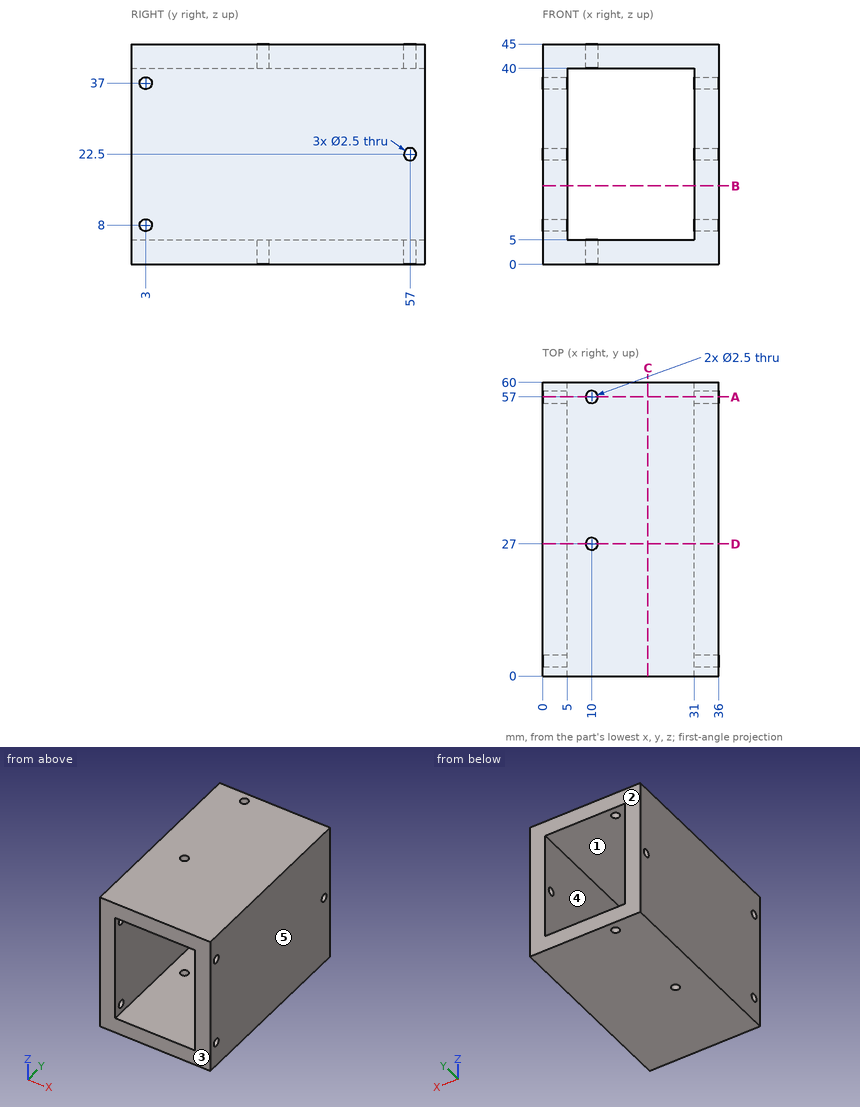
Here's the drawing with two shaded views (mm, measured from the low corner). I have some questions. A direction names the side the tool comes from. Give positions to 0.01 mm unless a question says otherwise; leave off trailing zeros. Order: outer loops, then holes, each group sorted by start corner. A loop starts at its lowest first (then second) coordinate and runs counter-clockwise, first axis right, second up.
Q1. If I drill on line 1 along X through (y, z) = (8, 9); line 2 along Z through (x, y) = (23, 24); line 3 along Y through (x, z) = (34, 8), over which ranges is the centre line in solid material (lowest first)?
Q2. We'd pull the mould along X, two halves only. Please class the marked faces 3, 4 and 5: +X half, -X half, draft (parallel to the pull), parting line (faces both ways), or undercut.
Q3. I'm going to push a flat-ended pin straight in: P1, Ø2, axis at y = 3, z = 37, coming from the -X side. Where does the tip first touch, or does it pass through?
Q4. Suppose I cut it at D-D, the plane y = 27. Write out the boundary of the cut face in (x, z), and give its area (3 significant figures).
Q5. For the marked faces 1 and 2, which set-ups out of +Z, -Z, +X, -X, +Y, -Y let a thin tool reach every point of the face, with its end or its side?
Q6. Suppose I cut it at C-C, the plane x = 21.5. Write out the boundary of the cut face in (y, z), and give its area (3 significant figures).
Q7. Suppose I cut it at B-B, the plane z = 16. Write out the boundary of the cut face in (x, y).
Q8. Suppose I cut it at A-A, the plane y = 57. Write out the boundary of the cut face in (x, z).
Solution:
1. line 1: x = 0 to 5, 31 to 36
1. line 2: z = 0 to 5, 40 to 45
1. line 3: y = 0 to 1.75, 4.25 to 60
2. face 3: draft
2. face 4: undercut
2. face 5: +X half
3. P1: passes through
4. outline: (0, 0) - (8.75, 0) - (8.75, 5) - (5, 5) - (5, 40) - (8.75, 40) - (8.75, 45) - (0, 45) - close; (11.25, 0) - (36, 0) - (36, 45) - (11.25, 45) - (11.25, 40) - (31, 40) - (31, 5) - (11.25, 5) - close
4. area: 685 mm2
5. face 1: +Y, -Y
5. face 2: +Z, -Z, +X, -X, +Y
6. outline: (0, 0) - (60, 0) - (60, 5) - (0, 5) - close; (0, 40) - (60, 40) - (60, 45) - (0, 45) - close
6. area: 600 mm2
7. outline: (0, 0) - (5, 0) - (5, 60) - (0, 60) - close; (31, 0) - (36, 0) - (36, 60) - (31, 60) - close
8. outline: (0, 0) - (8.75, 0) - (8.75, 5) - (5, 5) - (5, 21.25) - (0, 21.25) - close; (0, 23.75) - (5, 23.75) - (5, 40) - (8.75, 40) - (8.75, 45) - (0, 45) - close; (11.25, 0) - (36, 0) - (36, 21.25) - (31, 21.25) - (31, 5) - (11.25, 5) - close; (11.25, 40) - (31, 40) - (31, 23.75) - (36, 23.75) - (36, 45) - (11.25, 45) - close
